```python
from build123d import *

# Parameters (mm, degrees)
SKETCH_1_W          = 23.8
SKETCH_1_H          = 21.65
SKETCH_1_W_2        = 32
SKETCH_1_H_2        = 1.5
EXTRUDE_1_DEPTH     = 11.5
SKETCH_2_R          = 1
SKETCH_2_W          = 1.2
SKETCH_2_H          = 1.2
CUT_EXTRUDE_1_DEPTH = 11.5
SKETCH_3_R          = 5.75
SKETCH_3_R_2        = 2.875
EXTRUDE_2_DEPTH     = 3.8
SKETCH_4_R          = 2.5
EXTRUDE_3_DEPTH     = 3.8
CHAMFER_1_SIZE      = 1
CHAMFER_2_SIZE      = 0.5
SKETCH_5_R          = 0.5
SKETCH_5_W          = 1.377901166
SKETCH_5_H          = 0.226119028
EXTRUDE_5_DEPTH     = 4


with BuildPart() as part:
    # Эскиз1 → Бобышка-Вытянуть1 (new body)
    with BuildSketch(Plane.XY):
        Rectangle(SKETCH_1_W, SKETCH_1_H)
        with Locations((0, 6.225)):
            Rectangle(SKETCH_1_W_2, SKETCH_1_H_2)
    extrude(amount=EXTRUDE_1_DEPTH)

    # Эскиз2 → Вырез-Вытянуть1 (cut)
    with BuildSketch(Plane(origin=(0, 6.975, 0), x_dir=(1, 0, 0), z_dir=(0, 1, 0))):
        with Locations((-14, -5.75)):
            Circle(SKETCH_2_R)
        with Locations((14, -5.75)):
            Circle(SKETCH_2_R)
        with Locations((-15.4, -5.75)):
            Rectangle(SKETCH_2_W, SKETCH_2_H)
        with Locations((15.4, -5.75)):
            Rectangle(SKETCH_2_W, SKETCH_2_H)
    extrude(amount=-CUT_EXTRUDE_1_DEPTH, mode=Mode.SUBTRACT)

    # Эскиз3 → Бобышка-Вытянуть2 (add)
    with BuildSketch(Plane(origin=(0, 10.825, 0), x_dir=(1, 0, 0), z_dir=(0, 1, 0))):
        with Locations((6.15, -5.75)):
            Circle(SKETCH_3_R)
        with Locations((0.4, -5.75)):
            Circle(SKETCH_3_R_2)
    extrude(amount=EXTRUDE_2_DEPTH)

    # Эскиз4 → Бобышка-Вытянуть3 (add)
    with BuildSketch(Plane(origin=(0, 14.625, 0), x_dir=(1, 0, 0), z_dir=(0, 1, 0))):
        with Locations(Location((6.15, -5.75, 0), (0, 0, 270))):
            Circle(SKETCH_4_R)
    extrude(amount=EXTRUDE_3_DEPTH)

    # Фаска1
    chamfer_1_edges = [part.edges().sort_by_distance(p)[0] for p in [
        (-16, 6.225, 11.5),
        (-16, 6.225, 0),
        (16, 6.225, 0),
        (16, 6.225, 11.5),
    ]]
    chamfer(chamfer_1_edges, length=CHAMFER_1_SIZE)

    # Фаска2
    # the kernel refuses this chamfer: 0.5 mm, written as the material it takes off along each edge
    with BuildSketch(Plane(origin=(11.566666667, -10.491666667, 0.333333333), x_dir=(0.7071067811865476, 0, 0.7071067811865475), z_dir=(0.5773502691896257, -0.5773502691896258, -0.5773502691896258)), Plane(origin=(-11.566666667, 10.491666667, 11.166666667), x_dir=(-0.7071067811865475, -0.7071067811865475, 0), z_dir=(-0.5773502691896258, 0.5773502691896258, 0.5773502691896258)), Plane(origin=(-11.566666667, -10.491666667, 0.333333333), x_dir=(0, -0.7071067811865476, 0.7071067811865475), z_dir=(-0.5773502691896257, -0.5773502691896257, -0.5773502691896258)), Plane(origin=(11.566666667, 10.491666667, 0.333333333), x_dir=(0, 0.7071067811865476, 0.7071067811865475), z_dir=(0.5773502691896257, 0.5773502691896257, -0.5773502691896258))) as chamfer_2_piece_1:
        Polygon((-0.353553391, -0.204124145), (0.353553391, -0.204124145), (0, 0.40824829), align=None)
    extrude(amount=0.635085296, mode=Mode.SUBTRACT)
    with BuildSketch(Plane(origin=(11.566666667, -10.491666667, 11.166666667), x_dir=(-0.7071067811865475, -0.7071067811865475, 0), z_dir=(0.5773502691896258, -0.5773502691896258, 0.5773502691896258)), Plane(origin=(11.566666667, 10.491666667, 11.166666667), x_dir=(0.7071067811865475, -0.7071067811865475, 0), z_dir=(0.5773502691896258, 0.5773502691896258, 0.5773502691896258)), Plane(origin=(-11.566666667, 10.491666667, 0.333333333), x_dir=(0, 0.7071067811865476, 0.7071067811865475), z_dir=(-0.5773502691896257, 0.5773502691896257, -0.5773502691896258)), Plane(origin=(-11.566666667, -10.491666667, 11.166666667), x_dir=(0, -0.7071067811865475, -0.7071067811865475), z_dir=(-0.5773502691896258, -0.5773502691896258, 0.5773502691896258))) as chamfer_2_piece_2:
        Polygon((-0.353553391, 0.204124145), (0.353553391, 0.204124145), (0, -0.40824829), align=None)
    extrude(amount=0.635085296, mode=Mode.SUBTRACT)
    with BuildSketch(Plane(origin=(11.9, -10.825, -1.285841494), x_dir=(0.027495876610585647, 0.9996219169112968, 0), z_dir=(0, 0, 1)), Plane(origin=(-11.9, -10.825, -1.285841494), x_dir=(0.9996219169112968, -0.027495876610585647, 0), z_dir=(0, 0, 1))) as chamfer_2_piece_3:
        Polygon((CHAMFER_2_SIZE * 0.999621916911, CHAMFER_2_SIZE * 0.0274958766106), (-CHAMFER_2_SIZE * 0.0274958766106, CHAMFER_2_SIZE * 0.999621916911), (0, 0), align=None)
    extrude(amount=14.071682988, mode=Mode.SUBTRACT)
    with BuildSketch(Plane(origin=(11.9, 10.825, 5.75), x_dir=(0.027495876610585647, -0.9996219169112968, 0), z_dir=(0, 0, 1))) as chamfer_2_piece_4_section:
        Polygon((CHAMFER_2_SIZE * 0.999621916911, -CHAMFER_2_SIZE * 0.0274958766106), (-CHAMFER_2_SIZE * 0.0274958766106, -CHAMFER_2_SIZE * 0.999621916911), (0, 0), align=None)
    chamfer_2_piece_4 = extrude(amount=7.035841494, mode=Mode.PRIVATE)
    chamfer_2_piece_4 = chamfer_2_piece_4 - Plane(origin=(6.15, 10.65169011, 5.75), x_dir=(1, 0, 0), z_dir=(0, -1, 0)) * Cylinder(5.75, 17, mode=Mode.PRIVATE)
    add(chamfer_2_piece_4, mode=Mode.SUBTRACT)
    with BuildSketch(Plane(origin=(-11.9, 10.825, -1.285841494), x_dir=(0.9996219169112968, 0.027495876610585647, 0), z_dir=(0, 0, 1))) as chamfer_2_piece_5:
        Polygon((CHAMFER_2_SIZE * 0.999621916911, -CHAMFER_2_SIZE * 0.0274958766106), (-CHAMFER_2_SIZE * 0.0274958766106, -CHAMFER_2_SIZE * 0.999621916911), (0, 0), align=None)
    extrude(amount=14.071682988, mode=Mode.SUBTRACT)
    with BuildSketch(Plane(origin=(-11.9, 5.475, 11.5), x_dir=(-0.027495876610585647, 0, -0.9996219169112968), z_dir=(0, -1, 0)), Plane(origin=(11.9, -12.110841494, 11.5), x_dir=(0.027495876610585647, 0, -0.9996219169112968), z_dir=(0, 1, 0)), Plane(origin=(-11.9, 5.475, 0), x_dir=(0.9996219169112968, 0, -0.02749587661058639), z_dir=(0, -1, 0)), Plane(origin=(11.9, -12.110841494, 0), x_dir=(-0.9996219169112968, 0, -0.02749587661058639), z_dir=(0, 1, 0))) as chamfer_2_piece_6:
        Polygon((CHAMFER_2_SIZE * 0.999621916911, CHAMFER_2_SIZE * 0.0274958766106), (-CHAMFER_2_SIZE * 0.0274958766106, CHAMFER_2_SIZE * 0.999621916911), (0, 0), align=None)
    extrude(amount=17.585841494, mode=Mode.SUBTRACT)
    with BuildSketch(Plane(origin=(-11.9, 12.110841494, 11.5), x_dir=(-0.027495876610585647, 0, -0.9996219169112968), z_dir=(0, -1, 0)), Plane(origin=(11.9, 6.975, 11.5), x_dir=(0.027495876610585647, 0, -0.9996219169112968), z_dir=(0, 1, 0)), Plane(origin=(-11.9, 12.110841494, 0), x_dir=(0.9996219169112968, 0, -0.02749587661058639), z_dir=(0, -1, 0)), Plane(origin=(11.9, 6.975, 0), x_dir=(-0.9996219169112968, 0, -0.02749587661058639), z_dir=(0, 1, 0))) as chamfer_2_piece_7:
        Polygon((CHAMFER_2_SIZE * 0.999621916911, CHAMFER_2_SIZE * 0.0274958766106), (-CHAMFER_2_SIZE * 0.0274958766106, CHAMFER_2_SIZE * 0.999621916911), (0, 0), align=None)
    extrude(amount=5.135841494, mode=Mode.SUBTRACT)
    with BuildSketch(Plane(origin=(6.15, 10.825, 11.5), x_dir=(0, 0.027495876610585647, -0.9996219169112968), z_dir=(-1, 0, 0))) as chamfer_2_piece_8_section:
        Polygon((CHAMFER_2_SIZE * 0.999621916911, CHAMFER_2_SIZE * 0.0274958766106), (-CHAMFER_2_SIZE * 0.0274958766106, CHAMFER_2_SIZE * 0.999621916911), (0, 0), align=None)
    chamfer_2_piece_8 = extrude(amount=19.335841494, mode=Mode.PRIVATE)
    chamfer_2_piece_8 = chamfer_2_piece_8 - Plane(origin=(6.15, 10.656558796, 5.75), x_dir=(1, 0, 0), z_dir=(0, -1, 0)) * Cylinder(5.75, 41, mode=Mode.PRIVATE)
    add(chamfer_2_piece_8, mode=Mode.SUBTRACT)
    with BuildSketch(Plane(origin=(-13.185841494, -10.825, 11.5), x_dir=(0, -0.027495876610585647, -0.9996219169112968), z_dir=(1, 0, 0)), Plane(origin=(-13.185841494, -10.825, 0), x_dir=(0, 0.9996219169112968, -0.02749587661058639), z_dir=(1, 0, 0))) as chamfer_2_piece_9:
        Polygon((CHAMFER_2_SIZE * 0.999621916911, CHAMFER_2_SIZE * 0.0274958766106), (-CHAMFER_2_SIZE * 0.0274958766106, CHAMFER_2_SIZE * 0.999621916911), (0, 0), align=None)
    extrude(amount=26.371682988, mode=Mode.SUBTRACT)
    with BuildSketch(Plane(origin=(6.150000032, 10.825, 0), x_dir=(0, -0.9996219169112968, -0.02749587661058639), z_dir=(-1, 0, 0))) as chamfer_2_piece_10_section:
        Polygon((CHAMFER_2_SIZE * 0.999621916911, CHAMFER_2_SIZE * 0.0274958766106), (-CHAMFER_2_SIZE * 0.0274958766106, CHAMFER_2_SIZE * 0.999621916911), (0, 0), align=None)
    chamfer_2_piece_10 = extrude(amount=19.335841526, mode=Mode.PRIVATE)
    chamfer_2_piece_10 = chamfer_2_piece_10 - Plane(origin=(6.15, 10.656558796, 5.75), x_dir=(1, 0, 0), z_dir=(0, -1, 0)) * Cylinder(5.75, 41, mode=Mode.PRIVATE)
    add(chamfer_2_piece_10, mode=Mode.SUBTRACT)
    with BuildSketch(Plane(origin=(13.185841494, 10.825, 0), x_dir=(0, -0.9996219169112968, -0.02749587661058639), z_dir=(-1, 0, 0))) as chamfer_2_piece_11_section:
        Polygon((CHAMFER_2_SIZE * 0.999621916911, CHAMFER_2_SIZE * 0.0274958766106), (-CHAMFER_2_SIZE * 0.0274958766106, CHAMFER_2_SIZE * 0.999621916911), (0, 0), align=None)
    chamfer_2_piece_11 = extrude(amount=7.035841462, mode=Mode.PRIVATE)
    chamfer_2_piece_11 = chamfer_2_piece_11 - Plane(origin=(6.15, 10.65169011, 5.75), x_dir=(1, 0, 0), z_dir=(0, -1, 0)) * Cylinder(5.75, 17, mode=Mode.PRIVATE)
    add(chamfer_2_piece_11, mode=Mode.SUBTRACT)
    with BuildSketch(Plane(origin=(13.185841494, 10.825, 11.5), x_dir=(0, -0.9996219169112968, 0.027495876610585647), z_dir=(-1, 0, 0))) as chamfer_2_piece_12_section:
        Polygon((CHAMFER_2_SIZE * 0.999621916911, -CHAMFER_2_SIZE * 0.0274958766106), (-CHAMFER_2_SIZE * 0.0274958766106, -CHAMFER_2_SIZE * 0.999621916911), (0, 0), align=None)
    chamfer_2_piece_12 = extrude(amount=7.035841494, mode=Mode.PRIVATE)
    chamfer_2_piece_12 = chamfer_2_piece_12 - Plane(origin=(6.15, 10.65169011, 5.75), x_dir=(1, 0, 0), z_dir=(0, -1, 0)) * Cylinder(5.75, 17, mode=Mode.PRIVATE)
    add(chamfer_2_piece_12, mode=Mode.SUBTRACT)
    with BuildSketch(Plane(origin=(11.9, 10.825, -1.285841494), x_dir=(0.027495876610585647, -0.9996219169112968, 0), z_dir=(0, 0, 1))) as chamfer_2_piece_13_section:
        Polygon((CHAMFER_2_SIZE * 0.999621916911, -CHAMFER_2_SIZE * 0.0274958766106), (-CHAMFER_2_SIZE * 0.0274958766106, -CHAMFER_2_SIZE * 0.999621916911), (0, 0), align=None)
    chamfer_2_piece_13 = extrude(amount=7.035841494, mode=Mode.PRIVATE)
    chamfer_2_piece_13 = chamfer_2_piece_13 - Plane(origin=(6.15, 10.65169011, 5.75), x_dir=(1, 0, 0), z_dir=(0, -1, 0)) * Cylinder(5.75, 17, mode=Mode.PRIVATE)
    add(chamfer_2_piece_13, mode=Mode.SUBTRACT)

    # Эскиз5 → Бобышка-Вытянуть5 (add)
    with BuildSketch(Plane(origin=(11.9, 0, 0), x_dir=(0, 0, -1), z_dir=(1, 0, 0))):
        with Locations((-5.75, -6.825)):
            Circle(SKETCH_5_R)
        with Locations((-4.75, -6.825)):
            Circle(SKETCH_5_R)
        with Locations((-6.75, -6.825)):
            Circle(SKETCH_5_R)
        with Locations((-5.75, -6.825)):
            Rectangle(SKETCH_5_W, SKETCH_5_H)
    extrude(amount=EXTRUDE_5_DEPTH)


solid = part.part
```
Input: part model. Units: mm. Frame: model coordinates. A direction names the side the tool comes from. Give positions to 0.01 mm unless a question says otherwise; leave off trailing zeros. Write each loop counter-clockwise with the first axis right and the second up, starting at its lowest first coordinate (ties: lowest second). Pieces come first, ordered by that corner, then holes. Notation, with made-up numbers: (56, 54) - (73, 54) arc R9 cw to (73, 64) - close; hole circle Ø6 at (31, -31.75). An arc over 180 degrees is marked (long way). Write item = value, one per line. Start each with the question number.
1) Cut plane B-B (x = 14). Return loops of the section in (y, z) (3 decimals).
2) Reachability of faces 1 (the face through (15, 6, 5.15)), 2 (the face through (13.872, -7.325, 5.759)), 3 (the face through (-2.474, 12.698, 5.677)), 4 (the face through (13.87, -6.85, 4.25)) from +Z, -Z, +X, -X, +Y, -Y: full face, straight path, thin tool, end or side. Return the list, or none.
3) Cut plane D-D (x = 0.4). Return loops of the section in (y, z) (3 decimals).
4) Material intervals for L1, parallel to Z at x = 14, y = 6.05; L2, parallel to X at y = -8.5, z = 1.75; L3, parallel to Y at x = -2, z = 9 (3 decimals), sorted ascending. Write a range as [from, to].
5) Cut plane C-C (y = 6.5). Return loops of the section in (x, z), and give its area (3 significant figures).
6) Pin query (flat end, axial travel): pin 1 (0.8 mm diameter, centred on y = -7, z = 6, fed in from +X); pin 2 (1.5 mm diameter, centred on y = -0.5, z = 7.5, fed in from -X); pin 3 (1.2 mm diameter, centred on x = 14, z = 5.75, fed in from +Y) (3 decimals); pin 4 (4 mm diameter, centred on x = 3, y = 12, fed in from +Z). Return the tip coordinate at first contact, or that it passes through.
7) Draft query along X for faces 5 (the face through (0, 0, 0)), 6 (the face through (13, 6.2, 5.7)), 7 (the face through (-11.9, 9, 6)). Return one class per face: pulls with the +X half, pulls with the -X half, needs draft (parallel to the pull), parting line crosses it, or undercut.
8) Cut plane A-A (x = -14). Return loops of the section in (y, z) (3 decimals), and give its area (4 significant figures).
Answers follow:
q1.outline = (-6.938, 5.237) arc R0.5 ccw (long way) to (-6.712, 5.237) - (-6.712, 5.263) arc R0.5 ccw to (-6.712, 6.237) - (-6.712, 6.263) arc R0.5 ccw (long way) to (-6.938, 6.263) - (-6.938, 6.237) arc R0.5 ccw to (-6.938, 5.263) - close; (5.475, 0) - (6.975, 0) - (6.975, 4.75) - (5.475, 4.75) - close; (5.475, 6.75) - (6.975, 6.75) - (6.975, 11.5) - (5.475, 11.5) - close
q2.face_1 = +X, +Y
q2.face_2 = +X, -Y
q2.face_3 = +Y
q2.face_4 = +X
q3.outline = (-10.825, 0.5) - (-10.325, 0) - (10.325, 0) - (10.825, 0.5) - (10.825, 2.875) - (14.625, 2.875) - (14.625, 8.625) - (10.825, 8.625) - (10.825, 11) - (10.325, 11.5) - (-10.325, 11.5) - (-10.825, 11) - close
q4.L1 = [0, 4.75], [6.75, 11.5]
q4.L2 = [-11.9, 11.9]
q4.L3 = [-10.825, 10.825]
q5.outline = (-16, 1) - (-15, 0) - (15, 0) - (16, 1) - (16, 5.15) - (14.8, 5.15) arc R1 cw (long way) to (14.8, 6.35) - (16, 6.35) - (16, 10.5) - (15, 11.5) - (-15, 11.5) - (-16, 10.5) - (-16, 6.35) - (-14.8, 6.35) arc R1 cw (long way) to (-14.8, 5.15) - (-16, 5.15) - close
q5.area = 357 mm^2
q6.pin_1 = 15.9
q6.pin_2 = -11.9
q6.pin_3 = -6.325
q6.pin_4 = 11.5
q7.face_5 = needs draft
q7.face_6 = undercut
q7.face_7 = pulls with the -X half
q8.outline = (5.475, 0) - (6.975, 0) - (6.975, 4.75) - (5.475, 4.75) - close; (5.475, 6.75) - (6.975, 6.75) - (6.975, 11.5) - (5.475, 11.5) - close
q8.area = 14.25 mm^2
